Could you check a few things on this model? Use its own coordinates, in mm. Face numbers are marked on the shaded views. A direction names the side the tool comes from. Coordinates: 2 decimals unless noted, no trailing zeros. Loops run counter-clockwise (first coordinate to the right, second up) from the corner with the lowest first, then second, coordinate; pieces in that order, holes last.
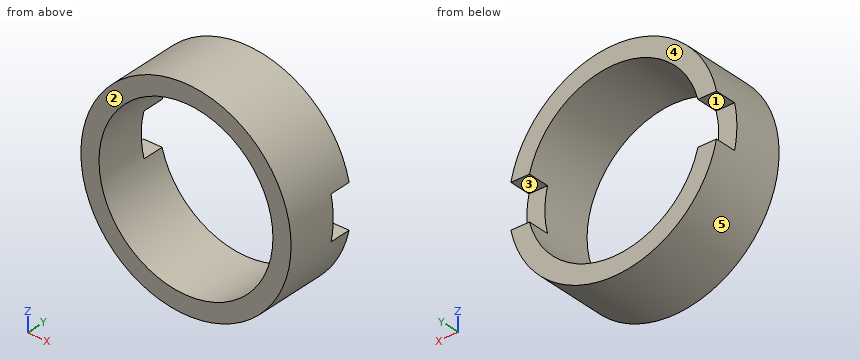
Autodesk Inventor part; units mm, degrees
ref_plane "YZ Plane" through (0, 0, 0) normal (1, 0, 0) x (0, 1, 0)
ref_plane "XZ Plane" through (0, 0, 0) normal (0, 1, 0) x (-1, 0, 0)
ref_plane "XY Plane" through (0, 0, 0) normal (0, 0, 1) x (1, 0, 0)
sketch "Esquisse1" plane through (0, 0, 0) normal (0, 1, 0) x (-1, 0, 0)
  circle A0 centre (0, 0) radius 7.25
  circle A1 centre (0, 0) radius 6
  dimension "d0" = 12
  dimension "d1" = 14.5
extrude "Extrusion1" add sketch "Esquisse1" along normal blind 5
sketch "Esquisse2" plane through (0, 5, 0) normal (0, 1, 0) x (1, 0, 0)
  line L0 (-8, -1.5) -> (-5, -1.5)
  line L1 (-5, -1.5) -> (-5, 1.5)
  line L2 (-5, 1.5) -> (-8, 1.5)
  line L3 (-8, 1.5) -> (-8, -1.5)
  line L4 (5, -1.5) -> (8, -1.5)
  line L5 (8, -1.5) -> (8, 1.5)
  line L6 (8, 1.5) -> (5, 1.5)
  line L7 (5, 1.5) -> (5, -1.5)
  point P0 (0, 0)
  dimension "d4" = 3
  dimension "d5" = 1.5
  dimension "d6" = 3
  dimension "d7" = 3
  dimension "d8" = 5
  dimension "d9" = 5
extrude "Extrusion2" cut sketch "Esquisse2" against normal blind 1.5
thread "Filetage1"
properties part number "Bague Prise Banane" material "Aluminium 6061"
(1) Imagine slicing it at C-C, the plane y = 2.9. Write out the boundary of the cut face in (x, z), and give its area (3 significant figures).
Answers:
outline: circle Ø14.5 at (0, 0); hole circle Ø12 at (0, 0)
area: 52.0 mm2
(2) Imagine slicing it at A-A, the plane x = 0. Write out the boundary of the cut face in (y, z), and give its area (3 significant figures).
Answers:
outline: (0, -7.25) - (5, -7.25) - (5, -6) - (0, -6) - close; (0, 6) - (5, 6) - (5, 7.25) - (0, 7.25) - close
area: 12.5 mm2
(3) For pin 1 (3 mm diameter, centred on x = -5.5, z = 3, fed in from -Y); pin 2 (1.5 mm diameter, centred on x = 2.5, y = 3.5, fed in from -Z); pin 3 (2 mm diameter, centred on x = 3, z = -3.5, fed in from +Y); pin 4 (1 mm diameter, centred on x = 6, y = 4.5, fed in from -Z), each with a flat end and sliding along its axis, tell me the tip position at first contact or that it passes through.
Answers:
pin 1: stops at y = 0
pin 2: stops at z = -7.04
pin 3: passes through
pin 4: stops at z = -4.72
(4) Which directions (+Z, -Z, +X, -X, +Y, -Y) give clear straight access to the entire face, cutting with the end or side of a thin tool? Please do the marked faces 1 and 2.
Answers:
face 1: +X, -X, +Y
face 2: +Z, -Z, +X, -X, -Y
(5) We'd pull the mould along Z, two halves only. Please class the marked faces 3, 4 and 5: +Z half, -Z half, draft (parallel to the pull), parting line (faces both ways), or undercut.
Answers:
face 3: undercut
face 4: draft
face 5: parting line
(6) I need wall thicknesses on probe 1 along Z at (x, y) = (0, 2.25); probe 2 along X at (y, z) = (2.75, -5.25). Which ranges of each line are inside material? Lowest first, please.
Answers:
probe 1: z = -7.25 to -6, 6 to 7.25
probe 2: x = -5 to -2.9, 2.9 to 5
(7) Imagine slicing it at B-B, the plane y = 3.8. Write out the boundary of the cut face in (x, z).
Answers:
outline: (-7.09, -1.5) arc R7.25 ccw to (7.09, -1.5) - (5.81, -1.5) arc R6 cw to (-5.81, -1.5) - close; (-7.09, 1.5) - (-5.81, 1.5) arc R6 cw to (5.81, 1.5) - (7.09, 1.5) arc R7.25 ccw to start
